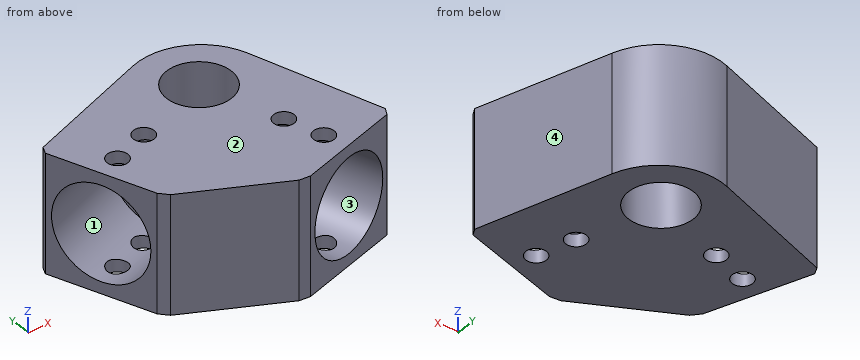
```python
from build123d import *

# Parameters (mm, degrees)
BOSS_EXTRUDE1_DEPTH = 40
SKETCH2_R           = 16
CUT_EXTRUDE1_DEPTH  = 30
SKETCH3_R           = 16
CUT_EXTRUDE2_DEPTH  = 30
CUT_EXTRUDE3_REACH  = 87.885
SKETCH4_R           = 3.5
SKETCH6_W           = 97.811122408
SKETCH6_H           = 40
BOSS_EXTRUDE2_DEPTH = 30
SKETCH5_R           = 11
CUT_EXTRUDE4_DEPTH  = 40
CUT_EXTRUDE7_DEPTH  = 40
FILLET1_R           = 22
CHAMFER1_SIZE       = 2
CHAMFER2_SIZE       = 2


with BuildPart() as part:
    # Sketch1 → Boss-Extrude1 (new body)
    with BuildSketch(Plane.XY):
        Polygon((-40.424029814, 28.51734538), (47.085187233, -15.176505431), (33.683689612, -42.016771106), (-53.825527435, 1.677079705), align=None)
        Polygon((-53.825527435, 1.677079705), (33.683689612, -42.016771106), (-4.585446216, -53.656068464), (-40.133712767, -35.906616376), align=None)
    extrude(amount=BOSS_EXTRUDE1_DEPTH)

    # Sketch2 → Cut-Extrude1 (cut)
    with BuildSketch(Plane(origin=(14.549121698, -47.836419785, 0), x_dir=(-0.9567283956954932, -0.29098243395423, 0), z_dir=(0.29098243395423, -0.9567283956954933, 0))):
        with Locations(Location((0, -20, 0), (0, 0, 180))):
            Circle(SKETCH2_R)
    extrude(amount=-CUT_EXTRUDE1_DEPTH, mode=Mode.SUBTRACT)

    # Sketch3 → Cut-Extrude2 (cut)
    with BuildSketch(Plane(origin=(-46.979620101, -17.114768336, 0), x_dir=(0, 0, 1), z_dir=(-0.939592402016652, -0.342295366712111, 0))):
        with Locations(Location((20, 0, 0), (0, 0, 270))):
            Circle(SKETCH3_R)
    extrude(amount=-CUT_EXTRUDE2_DEPTH, mode=Mode.SUBTRACT)

    # Cut-Extrude3: up to this face of the body (flat: up to its plane)
    cut_extrude3_end = Plane(part.part.faces().sort_by_distance((-8.066388037, -16.155209221, 40))[0])
    # Sketch4 → Cut-Extrude3 (cut, up to the picked face)
    with BuildSketch(Plane(origin=(0, 0, 0), x_dir=(-1, 0, 0), z_dir=(0, 0, -1)), mode=Mode.PRIVATE) as cut_extrude3_sk1:
        with Locations((-8.241246184, -27.096598695)):
            Circle(SKETCH4_R)
    cut_extrude3_tool1 = split(extrude(cut_extrude3_sk1.sketch, amount=-CUT_EXTRUDE3_REACH, mode=Mode.PRIVATE), bisect_by=cut_extrude3_end, keep=Keep.BOTH, mode=Mode.PRIVATE)
    # Sketch4 → Cut-Extrude3 (cut, up to the picked face)
    with BuildSketch(Plane(origin=(0, 0, 0), x_dir=(-1, 0, 0), z_dir=(0, 0, -1)), mode=Mode.PRIVATE) as cut_extrude3_sk2:
        with Locations((-12.125238023, -39.866872249)):
            Circle(SKETCH4_R)
    cut_extrude3_tool2 = split(extrude(cut_extrude3_sk2.sketch, amount=-CUT_EXTRUDE3_REACH, mode=Mode.PRIVATE), bisect_by=cut_extrude3_end, keep=Keep.BOTH, mode=Mode.PRIVATE)
    # Sketch4 → Cut-Extrude3 (cut, up to the picked face)
    with BuildSketch(Plane(origin=(0, 0, 0), x_dir=(-1, 0, 0), z_dir=(0, 0, -1)), mode=Mode.PRIVATE) as cut_extrude3_sk3:
        with Locations((26.555072549, -9.674065347)):
            Circle(SKETCH4_R)
    cut_extrude3_tool3 = split(extrude(cut_extrude3_sk3.sketch, amount=-CUT_EXTRUDE3_REACH, mode=Mode.PRIVATE), bisect_by=cut_extrude3_end, keep=Keep.BOTH, mode=Mode.PRIVATE)
    # Sketch4 → Cut-Extrude3 (cut, up to the picked face)
    with BuildSketch(Plane(origin=(0, 0, 0), x_dir=(-1, 0, 0), z_dir=(0, 0, -1)), mode=Mode.PRIVATE) as cut_extrude3_sk4:
        with Locations((39.152815392, -14.263447931)):
            Circle(SKETCH4_R)
    cut_extrude3_tool4 = split(extrude(cut_extrude3_sk4.sketch, amount=-CUT_EXTRUDE3_REACH, mode=Mode.PRIVATE), bisect_by=cut_extrude3_end, keep=Keep.BOTH, mode=Mode.PRIVATE)
    add(cut_extrude3_tool1.solids().sort_by(Axis((8.241246, -27.096599, 0), (0, 0, 1)))[0], mode=Mode.SUBTRACT)
    add(cut_extrude3_tool2.solids().sort_by(Axis((12.125238, -39.866872, 0), (0, 0, 1)))[0], mode=Mode.SUBTRACT)
    add(cut_extrude3_tool3.solids().sort_by(Axis((-26.555073, -9.674065, 0), (0, 0, 1)))[0], mode=Mode.SUBTRACT)
    add(cut_extrude3_tool4.solids().sort_by(Axis((-39.152815, -14.263448, 0), (0, 0, 1)))[0], mode=Mode.SUBTRACT)

    # Sketch6 → Boss-Extrude2 (add)
    with BuildSketch(Plane(origin=(3.33057871, 6.670419974, 0), x_dir=(0.8946755224974542, -0.4467165873838887, 0), z_dir=(0.4467165873838887, 0.8946755224974542, 0))):
        with Locations((0, -20)):
            Rectangle(SKETCH6_W, SKETCH6_H)
    extrude(amount=BOSS_EXTRUDE2_DEPTH)

    # Sketch5 → Cut-Extrude4 (cut)
    with BuildSketch(Plane(origin=(0, 0, 0), x_dir=(-1, 0, 0), z_dir=(0, 0, -1))):
        Circle(SKETCH5_R)
    extrude(amount=-CUT_EXTRUDE4_DEPTH, mode=Mode.SUBTRACT)

    # Sketch7 → Cut-Extrude7 (cut)
    with BuildSketch(Plane(origin=(0, 0, 0), x_dir=(-1, 0, 0), z_dir=(0, 0, -1))):
        Polygon((-60.486684855, 11.663760244), (-33.683689612, -42.016771106), (-12.991209784, 26.018548963), (-23.829432932, 29.966935049), align=None)
        Polygon((-23.829432932, 29.966935049), (-12.991209784, 26.018548963), (-9.634719731, 37.05443625), align=None)
        Polygon((-9.634719731, 37.05443625), (-12.991209784, 26.018548963), (53.825527435, 1.677079705), (27.022532192, 55.357611055), align=None)
    extrude(amount=-CUT_EXTRUDE7_DEPTH, mode=Mode.SUBTRACT)

    # Fillet1
    fillet1_edges = [part.edges().sort_by_distance(p)[0] for p in [
        (12.991209784, 26.018548963, 20),
    ]]
    fillet(fillet1_edges, radius=FILLET1_R)

    # Chamfer1
    chamfer1_edges = [part.edges().sort_by_distance(p)[0] for p in [
        (33.683689612, -42.016771106, 20),
        (-53.825527435, 1.677079705, 20),
    ]]
    chamfer(chamfer1_edges, length=CHAMFER1_SIZE)

    # Chamfer2
    chamfer2_edges = [part.edges().sort_by_distance(p)[0] for p in [
        (-4.585446216, -53.656068464, 20),
        (-40.133712767, -35.906616376, 20),
    ]]
    chamfer(chamfer2_edges, length=CHAMFER2_SIZE)


solid = part.part
```
Could you check a few things on this model? Use its own coordinates, in mm. Face numbers are marked on the shaded views. Coordinates: 2 decimals unless noted, no trailing zeros. Write each loop counter-clockwise with the first axis right and the second up, starting at its lowest first coordinate (ties: lowest second). Pieces come first, ordered by that corner, then holes. Notation, with made-up numbers: (80, 56) -> (109, 56) arc R15 ccw to (109, 78) -> close; hole circle Ø7 at (14, 48). An arc over 180 degrees is marked (long way). One line per question, with ' | ' between items. Start each with the question number.
1. Please list where these lines run through material, in increasing order: line 1 along X through (y, z) = (-32, 25); line 2 along X through (y, z) = (-41, 30); line 3 along Y through (x, z) = (4, 11).
2. If we section it at C-C (z = 24.5): Please give me the cut outline in (x, y), and give its area (3 significant figures).
3. Thinking about a two-plate mould opening in Z: for the marked faces 1, 2, 3 and 4, which applies, pulls with the +Z half, pulls with the -Z half, needs draft (parallel to the pull), parting line crosses it, or undercut?
4. If we section it at A-A (z = 10.5): Please give me the cut outline in (x, y) (3 decimals).
5. Will these pins go through, and if not, where does the flat tip stop? P1, Ø2, axis at y = -19, z = 24, coming from the -X side; P2, Ø11, axis at x = 8.24, y = -27.1, coming from the -Z side; P3, Ø4, axis at x = 8.24, y = -27.1, coming from the -Z side; P4, Ø5, axis at y = -32.5, z = 27.5, coming from the +X side.
6. If we section it at B-B (y = -8): Count the separate pieces of the cut face and the enclosed holes in it, and give its area (3 significant figures).
Return value:
1) line 1: x = -41.56 to -6.15, 25.62 to 30.64 | line 2: x = -29.93 to -0.59, 25.52 to 32.62 | line 3: y = -19.69 to -10.25, 10.25 to 18.75
2) outline: (-53.14, -0.2) -> (-52.24, -2.69) -> (-24.05, 7.58) -> (-13.54, -21.27) -> (-41.72, -31.54) -> (-40.82, -34.03) -> (-38.34, -36.8) -> (-6.37, -52.76) -> (-2.67, -53.07) -> (-0.14, -52.3) -> (-8.87, -23.6) -> (20.51, -14.67) -> (29.24, -43.37) -> (31.77, -42.6) -> (33.1, -40.1) -> (19.75, 3.8) arc R22 ccw to (-8.83, 18.07) -> (-51.95, 2.36) -> close; hole circle Ø22 at (0, 0) | area: 2,070 mm²
3) face 1: undercut | face 2: pulls with the +Z half | face 3: undercut | face 4: needs draft
4) outline: (-53.141, -0.202) -> (-51.386, -5.018) -> (-23.199, 5.251) -> (-14.385, -18.943) -> (-42.573, -29.211) -> (-40.818, -34.027) -> (-38.344, -36.8) -> (-6.375, -52.763) -> (-2.672, -53.074) -> (2.232, -51.583) -> (-6.498, -22.881) -> (18.137, -15.388) -> (26.866, -44.09) -> (31.77, -42.599) -> (33.102, -40.103) -> (19.749, 3.8) arc R22 ccw to (-8.83, 18.069) -> (-51.946, 2.362) -> close; hole circle Ø22 at (0, 0)
5) P1: stops at x = -14.73 | P2: stops at z = 0 | P3: passes through | P4: stops at x = 31.55
6) separate pieces: 4 | enclosed holes: 0 | area: 1,330 mm²
